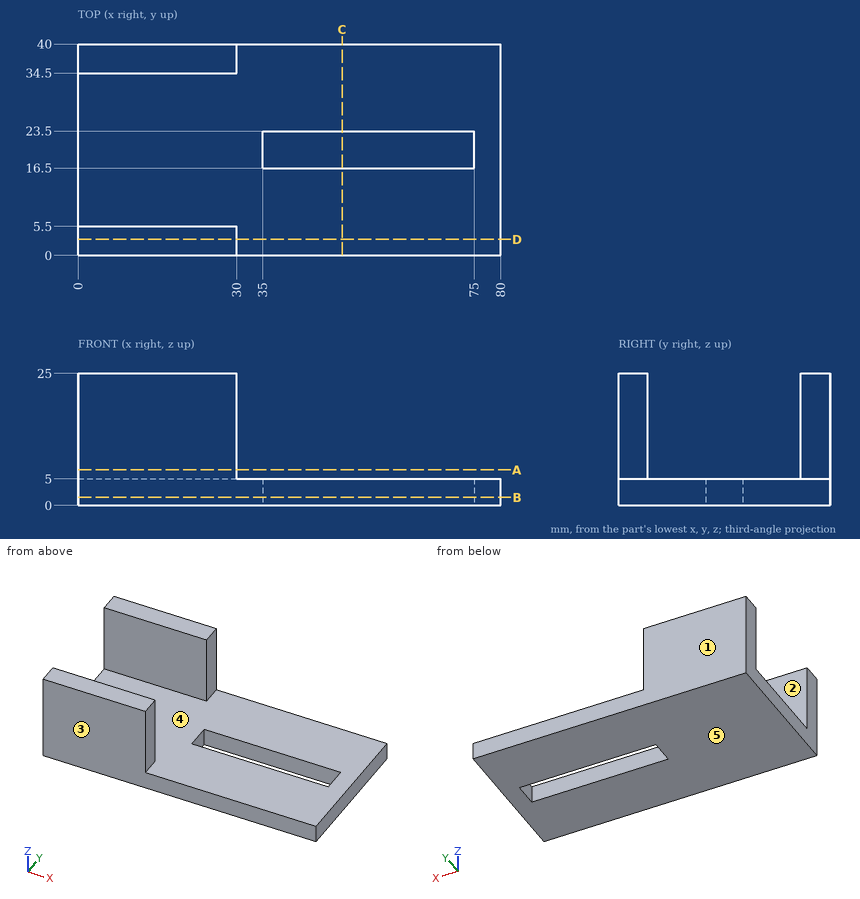
Geometry: see drawing. Coordinates: mm, zero at the bounding-box minimum. A direction names the side the tool comes from. Coordinates: 2 decimals unless noted, no trailing zeros. Loops run counter-clockwise (first coordinate to the right, second up) from the corner with the lowest first, then second, coordinate; pieces in that order, holes last. Notation, with made-up numbers: (-25, 1) - (-21, 1) arc R34 cw to (-21, 36) - close; hole circle Ø8 at (56.5, 46.25). An arc over 180 degrees is marked (long way). Answer as CSV lines item,"result".
1. Section A-A (z = 6.75). Return loops of the section in (x, y), then the cut area to 3 significant figures.
Established:
outline,"(0, 0) - (30, 0) - (30, 5.5) - (0, 5.5) - close; (0, 34.5) - (30, 34.5) - (30, 40) - (0, 40) - close"
area,"330 mm2"
2. Reachability of the marked faces 1 and 2 from +Z, -Z, +X, -X, +Y, -Y: full face, straight path, thin tool, end or side. Return the list, or none.
Established:
face 1,"+Z, -Z, +X, -X, +Y"
face 2,"+Z, +X, -X"
3. Contact query for flat-ended pins moving along their axis: pin 1 (12 mm diameter, centred on x = 39, y = 24, fed in from +Z); pin 2 (1.6 mm diameter, centred on y = 3, z = 14.5, fed in from +X). Output: stop coordinate, or through.
Established:
pin 1,"stops at z = 5"
pin 2,"stops at x = 30"
4. Section C-C (x = 50). Return loops of the section in (y, z).
Established:
outline,"(0, 0) - (16.5, 0) - (16.5, 5) - (0, 5) - close; (23.5, 0) - (40, 0) - (40, 5) - (23.5, 5) - close"
5. Mould query, pull axis Y, two halves, no side actions, for the marked faces 3, 4 and 5. Classes: released by +Y, released by -Y, zero draft, split by the parting line, or undercut.
Established:
face 3,"released by -Y"
face 4,"undercut"
face 5,"zero draft"
6. Ray query, line 1 (Y direction, x = 26.5, z = 11.5); line 2 (X direction, y = 22, z = 2); line 3 (Z direction, x = 59, y = 29). Return the intervals inside material, ascending.
Established:
line 1,"y = 0 to 5.5, 34.5 to 40"
line 2,"x = 0 to 35, 75 to 80"
line 3,"z = 0 to 5"
7. Section D-D (y = 3). Return loops of the section in (x, z), then the cut area to 3 significant figures.
Established:
outline,"(0, 0) - (80, 0) - (80, 5) - (30, 5) - (30, 25) - (0, 25) - close"
area,"1,000 mm2"
8. Section B-B (z = 1.5). Return loops of the section in (x, y), then the cut area to 3 significant figures.
Established:
outline,"(0, 0) - (80, 0) - (80, 40) - (0, 40) - close; hole (35, 16.5) - (75, 16.5) - (75, 23.5) - (35, 23.5) - close"
area,"2,920 mm2"
